```python
from build123d import *

# Parameters (mm, degrees)
SKETCH1_W             = 29.8
SKETCH1_H             = 29.8
BOSS_EXTRUDE1_DEPTH   = 6.35
BOSS_EXTRUDE1_2_DEPTH = 6.35
BOSS_EXTRUDE1_3_DEPTH = 6.35
BOSS_EXTRUDE1_4_DEPTH = 6.35
SKETCH2_W             = 79.8
SKETCH2_H             = 79.8
BOSS_EXTRUDE2_DEPTH   = 8
FILLET2_R             = 10
SKETCH3_R             = 35
SKETCH3_R_2           = 30
BOSS_EXTRUDE3_DEPTH   = 30
FILLET3_R             = 30
FILLET4_R             = 1
SKETCH4_R             = 2.125
CUT_EXTRUDE1_DEPTH    = 5
SKETCH6_R             = 5
CUT_EXTRUDE2_DEPTH    = 30
SKETCH7_R             = 1.75
CUT_EXTRUDE3_DEPTH    = 100.337908172
SKETCH8_R             = 3
CUT_EXTRUDE4_DEPTH    = 4


with BuildPart() as part:
    # Sketch1 → Boss-Extrude1 (new body)
    with BuildSketch(Plane.XY):
        Rectangle(SKETCH1_W, SKETCH1_H)
    extrude(amount=BOSS_EXTRUDE1_DEPTH)



with BuildPart() as body_2:
    # Sketch1 → Boss-Extrude1 2 (new body)
    with BuildSketch(Plane.XY):
        with Locations((50, 0)):
            Rectangle(SKETCH1_W, SKETCH1_H)
    extrude(amount=BOSS_EXTRUDE1_2_DEPTH)


with BuildPart() as body_3:
    # Sketch1 → Boss-Extrude1 3 (new body)
    with BuildSketch(Plane.XY):
        with Locations((50, 50)):
            Rectangle(SKETCH1_W, SKETCH1_H)
    extrude(amount=BOSS_EXTRUDE1_3_DEPTH)


with BuildPart() as body_4:
    # Sketch1 → Boss-Extrude1 4 (new body)
    with BuildSketch(Plane.XY):
        with Locations((0, 50)):
            Rectangle(SKETCH1_W, SKETCH1_H)
    extrude(amount=BOSS_EXTRUDE1_4_DEPTH)


with BuildPart() as part_1:
    add(part.part)

    add(body_2.part)  # Boss-Extrude2 merges body 2

    add(body_3.part)  # Boss-Extrude2 merges body 3

    add(body_4.part)  # Boss-Extrude2 merges body 4
    # Sketch2 → Boss-Extrude2 (add)
    with BuildSketch(Plane.XY.offset(6.35)):
        with Locations((25, 25)):
            Rectangle(SKETCH2_W, SKETCH2_H)
    extrude(amount=BOSS_EXTRUDE2_DEPTH)

    # Fillet2
    fillet2_edges = [part_1.edges().sort_by_distance(p)[0] for p in [
        (-14.9, 64.9, 7.175),
        (64.9, -14.9, 7.175),
        (64.9, 64.9, 7.175),
        (35.1, 14.9, 3.175),
        (35.1, -14.9, 3.175),
        (64.9, 14.9, 3.175),
        (35.1, 64.9, 3.175),
        (35.1, 35.1, 3.175),
        (64.9, 35.1, 3.175),
        (-14.9, 35.1, 3.175),
        (14.9, 35.1, 3.175),
        (14.9, 64.9, 3.175),
        (-14.9, 14.9, 3.175),
        (14.9, 14.9, 3.175),
        (14.9, -14.9, 3.175),
        (-14.9, -14.9, 7.175),
    ]]
    fillet(fillet2_edges, radius=FILLET2_R)

    # Sketch3 → Boss-Extrude3 (add)
    with BuildSketch(Plane.XY.offset(14.35)):
        with Locations(Location((25, 25, 0), (0, 0, 180))):
            Circle(SKETCH3_R)
        with Locations((25, 25)):
            Circle(SKETCH3_R_2, mode=Mode.SUBTRACT)
    extrude(amount=BOSS_EXTRUDE3_DEPTH)

    # Fillet3
    fillet3_edges = [part_1.edges().sort_by_distance(p)[0] for p in [
        (-5, 25, 14.35),
    ]]
    fillet(fillet3_edges, radius=FILLET3_R - 0.0001)  # a hair under: the kernel refuses the full size

    # Fillet4
    fillet4_edges = [part_1.edges().sort_by_distance(p)[0] for p in [
        (60, 25, 44.35),
    ]]
    fillet(fillet4_edges, radius=FILLET4_R)

    # Sketch4 → Cut-Extrude1 (cut)
    with BuildSketch(Plane(origin=(0, 0, 0), x_dir=(-1, 0, 0), z_dir=(0, 0, -1))):
        with Locations((0, 50)):
            Circle(SKETCH4_R)
        Circle(SKETCH4_R)
        with Locations((-50, 0)):
            Circle(SKETCH4_R)
        with Locations((-50, 50)):
            Circle(SKETCH4_R)
    extrude(amount=-CUT_EXTRUDE1_DEPTH, mode=Mode.SUBTRACT)

    # Sketch6 → Cut-Extrude2 (cut)
    with BuildSketch(Plane.XY.offset(44.35)):
        with Locations((25, 25)):
            Circle(SKETCH6_R)
    extrude(amount=-CUT_EXTRUDE2_DEPTH, mode=Mode.SUBTRACT)

    # Sketch7 → Cut-Extrude3 (cut, through all)
    with BuildSketch(Plane(origin=(0, 0, 6.35), x_dir=(-1, 0, 0), z_dir=(0, 0, -1))):
        with Locations((-25, 25)):
            Circle(SKETCH7_R)
    extrude(amount=-CUT_EXTRUDE3_DEPTH, mode=Mode.SUBTRACT)

    # Sketch8 → Cut-Extrude4 (cut)
    with BuildSketch(Plane(origin=(0, 0, 6.35), x_dir=(-1, 0, 0), z_dir=(0, 0, -1))):
        with Locations((-25, 25)):
            Circle(SKETCH8_R)
    extrude(amount=-CUT_EXTRUDE4_DEPTH, mode=Mode.SUBTRACT)


solid = part_1.part
```
For this review, take the finished solid that the model builds, in its own axes (mm). A direction names the side the tool comes from. Round coordinates to 2 decimals unless told otherwise and drop trailing zeros. Loops run counter-clockwise (first coordinate to the right, second up) from the corner with the lowest first, then second, coordinate; pieces in that order, holes last.
Q1. Mouldability with a two-part tool opening along X and no side actions: class faces 4 (the face through (0, -3, 0)), 5 (the face through (-12.05, 61.89, 7.07)), 6 (the face through (35.1, 0, 3)), 7 (the face through (8.85, 56.05, 28.65)) as +X half, -X half, draft (parallel to the pull), parting line (faces both ways), or undercut.
Result sheet:
face 4: draft
face 5: -X half
face 6: undercut
face 7: parting line
Q2. Add section A-A on z = 7.5. Write out the cut boundary in (x, y), plus the area to 3 significant figures.
Result sheet:
outline: (-14.9, -4.9) arc R10 ccw to (-4.9, -14.9) - (54.9, -14.9) arc R10 ccw to (64.9, -4.9) - (64.9, 54.9) arc R10 ccw to (54.9, 64.9) - (-4.9, 64.9) arc R10 ccw to (-14.9, 54.9) - close; hole circle Ø6 at (25, 25)
area: 6,250 mm2
Q3. To check wall thickness, follow line 1 along Y through (x, z) = (50, 1) (3 decimals). State the ranges of the line that lie inside material, in increasing order.
Result sheet:
line 1: y = -14.9 to -2.125, 2.125 to 14.9, 35.1 to 47.875, 52.125 to 64.9
Q4. Machinability: for faces 1 (the face through (12.05, 61.89, 3.22)), 2 (the face through (11.89, -12.05, 3.22)), 3 (the face through (0, 0, 5)), which of the approach directions +Z, -Z, +X, -X, +Y, -Y give a long, thin tool a straight path to every point of the face, cutting with its end or side? Answer none if there is none.
Result sheet:
face 1: -Z, +Y
face 2: -Z, -Y
face 3: -Z
Q5. Insertion check: pin 1 Ø1 at (x, z) = (23, 28) entering from +Y; pin 2 Ø2 at (x, y) = (49.5, 50) entering from -Z; pin 3 Ø2 at (x, z) = (18.5, 19.5) entering from -Y. Each pin has a flat end and moves straight along its axis. Give the tip position at first contact, or say it passes through.
Result sheet:
pin 1: stops at y = 59.97
pin 2: stops at z = 5
pin 3: stops at y = -9.57
